Verification items for this drawing (mm, ordinates from the low corner). A direction names the side the tool comes from. Round coordinates to 2 decimals unless told otherwise and drop trailing zeros. Order: outer loops, then holes, each group sorted by start corner. A loop starts at its lowest first (then second) coordinate and runs counter-clockwise, first axis right, second up. Notation, with made-up numbers: (43.5, 6) - (99.5, 6) arc R15 cw to (99.5, 26) - close; hole circle Ø1 at (-15.75, 38). An arc over 180 degrees is marked (long way). Use a Markdown table: item, result. Add a question column.
(1) Thickness scan on line 1 along Y through (x, z) = (35.25, 2.95); line 2 along X through (y, z) = (2, 14); line 3 along Y through (x, z) = (23, 19.5). Record the ranges inside material, lowest first. Write a range as [from, to].
(2) Access from +Z, -Z, +X, -X, +Y, -Y to the whole of each face (thin tool, end or side, straight path). Record for the marked faces 5 and 6.
(3) Mould release check, pull along Y, two halves, no side actions. Record for the marked faces 1, 2, 3 and 4: released by +Y, released by -Y, zero draft, split by the parting line, or undercut.
(4) Section check A-A on x = 25. Record the boundary of the cut face in (y, z).
(5) Section check C-C on x = 40. Record the boundary of the cut face in (y, z), then the cut area to 3 significant figures.
(6) Section check B-B on z = 14. Record the boundary of the cut face in (x, y).
(7) Section check D-D on z = 7.75. Record the boundary of the cut face in (x, y), then the cut area to 3 significant figures.
(8) Gauge pin test, flat ends, axial feed: P1, Ø4, axis at x = 40, z = 14, coming from the +Y side; P2, Ø4.5, axis at x = 14.75, y = 16.75, coming from the +Z side; P3, Ø5, axis at x = 40, z = 14, coming from the -Y side. Record the tip position at first contact, or that the pin passes through.
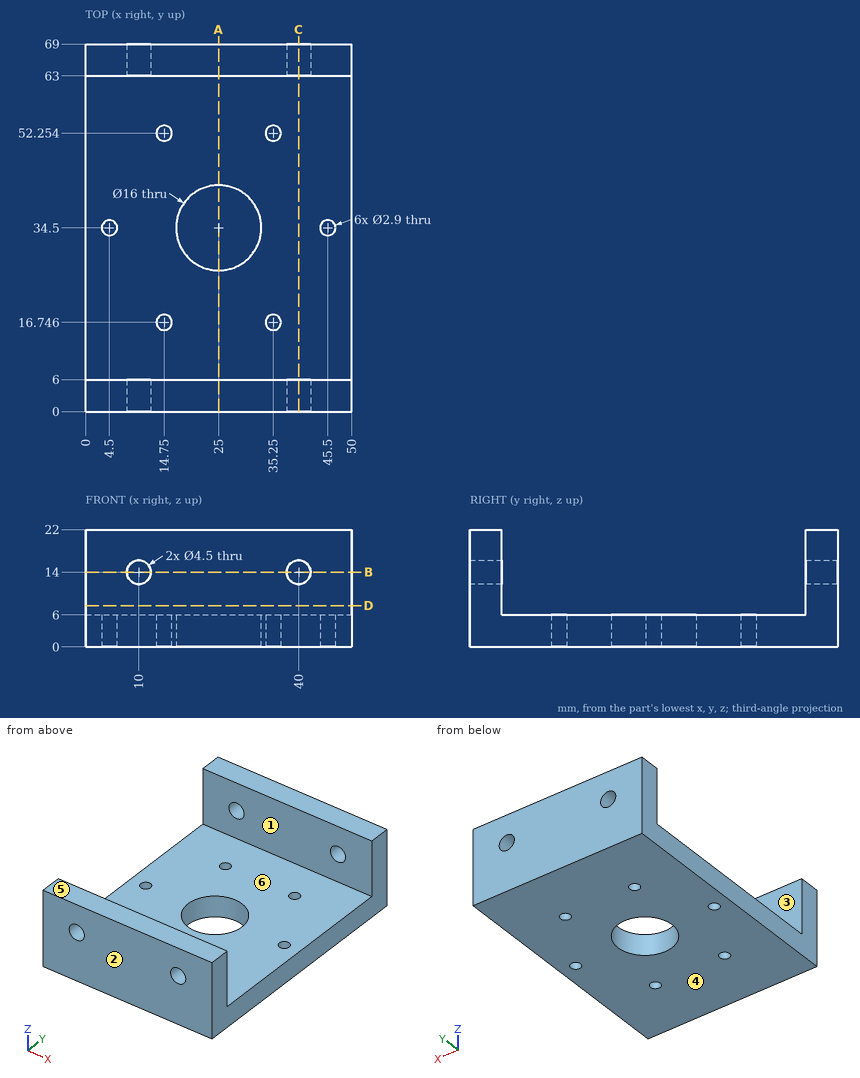
Check sheet entries:
| question | item | result |
|---|---|---|
| 1 | line 1 | y = [0, 15.3], [18.2, 50.8], [53.7, 69] |
| 1 | line 2 | x = [0, 7.75], [12.25, 37.75], [42.25, 50] |
| 1 | line 3 | y = [0, 6], [63, 69] |
| 2 | face 5 | +Z, +X, -X, +Y, -Y |
| 2 | face 6 | +Z, +X, -X |
| 3 | face 1 | undercut |
| 3 | face 2 | released by -Y |
| 3 | face 3 | undercut |
| 3 | face 4 | zero draft |
| 4 | outline | (0, 0) - (26.5, 0) - (26.5, 6) - (6, 6) - (6, 22) - (0, 22) - close; (42.5, 0) - (69, 0) - (69, 22) - (63, 22) - (63, 6) - (42.5, 6) - close |
| 5 | outline | (0, 0) - (69, 0) - (69, 11.75) - (63, 11.75) - (63, 6) - (6, 6) - (6, 11.75) - (0, 11.75) - close; (0, 16.25) - (6, 16.25) - (6, 22) - (0, 22) - close; (63, 16.25) - (69, 16.25) - (69, 22) - (63, 22) - close |
| 5 | area | 552 mm2 |
| 6 | outline | (0, 0) - (7.75, 0) - (7.75, 6) - (0, 6) - close; (0, 63) - (7.75, 63) - (7.75, 69) - (0, 69) - close; (12.25, 0) - (37.75, 0) - (37.75, 6) - (12.25, 6) - close; (12.25, 63) - (37.75, 63) - (37.75, 69) - (12.25, 69) - close; (42.25, 0) - (50, 0) - (50, 6) - (42.25, 6) - close; (42.25, 63) - (50, 63) - (50, 69) - (42.25, 69) - close |
| 7 | outline | (0, 0) - (50, 0) - (50, 6) - (0, 6) - close; (0, 63) - (50, 63) - (50, 69) - (0, 69) - close |
| 7 | area | 600 mm2 |
| 8 | P1 | passes through |
| 8 | P2 | stops at z = 6 |
| 8 | P3 | stops at y = 0 |
